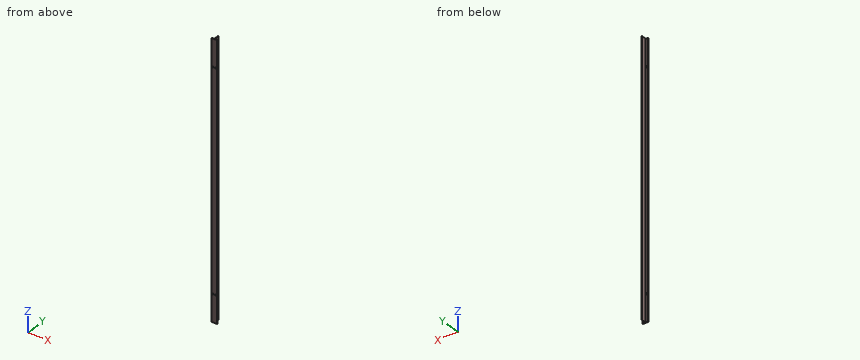
from build123d import *

# Parameters (mm, degrees)
EXTRUDE_1_DEPTH     = 1000
SKETCH_2_R          = 2
CUT_EXTRUDE_1_DEPTH = 10


with BuildPart() as part:
    # Эскиз1 → Бобышка-Вытянуть1 (new body)
    with BuildSketch(Plane.XY):
        Polygon((0.75, 20), (-0.75, 20), (-0.75, 1.5), (-10, 1.5), (-10, 0), (10, 0), (10, 1.5), (0.75, 1.5), align=None)
    extrude(amount=EXTRUDE_1_DEPTH)

    # Эскиз2 → Вырез-Вытянуть1 (cut)
    with BuildSketch(Plane.XZ):
        with Locations(Location((5, 900, 0), (0, 0, 270))):
            Circle(SKETCH_2_R)
        with Locations(Location((-5, 900, 0), (0, 0, 270))):
            Circle(SKETCH_2_R)
        with Locations((5, 100)):
            Circle(SKETCH_2_R)
        with Locations((-5, 100)):
            Circle(SKETCH_2_R)
    extrude(amount=-CUT_EXTRUDE_1_DEPTH, mode=Mode.SUBTRACT)


solid = part.part
Part model, mm, in its own coordinate system. Give positions to 0.01 mm unless a question says otherwise; leave off trailing zeros. Loops run counter-clockwise (first coordinate to the right, second up) from the corner with the lowest first, then second, coordinate; pieces in that order, holes last.
(1) Pin check, flat tips, straight feed: pin 1 (10 mm diameter, centred on x = -6.5, z = 399.5, fed in from +Y); pin 2 (4 mm diameter, centred on x = 4, y = 10.5, fed in from +Z); pin 3 (5.5 mm diameter, centred on y = 12, z = 515.5, fed in from -X). Stop position of each tip, or through.
Return value:
pin 1: stops at y = 1.5
pin 2: passes through
pin 3: stops at x = -0.75
(2) Band-saw the part on B-B (y = 12.5). Write the cut outline in (x, z).
Return value:
outline: (-0.75, 0) - (0.75, 0) - (0.75, 1000) - (-0.75, 1000) - close
(3) Drill centre lines: line 1 along X through (y, z) = (0.7, 900); line 2 along X through (y, z) = (13, 489); line 3 along Y through (x, z) = (-1.75, 464). Where is each one in solid material? Low to high.
Return value:
line 1: x = -10 to -7, -3 to 3, 7 to 10
line 2: x = -0.75 to 0.75
line 3: y = 0 to 1.5
(4) Band-saw the part on A-A (z = 532). Write the cut outline in (x, y), and give its area (4 significant figures).
Return value:
outline: (-10, 0) - (10, 0) - (10, 1.5) - (0.75, 1.5) - (0.75, 20) - (-0.75, 20) - (-0.75, 1.5) - (-10, 1.5) - close
area: 57.75 mm2
